Geometry check sheet. Reference: the model listing, model coordinates, mm. Face numbers are marked on the shaded views. A direction names the side the tool comes from. Give positions to 0.01 mm unless a question says otherwise; leave off trailing zeros. Write each loop counter-clockwise with the first axis right and the second up, starting at its lowest first coordinate (ties: lowest second). Pieces come first, ordered by that corner, then holes. Notation, with made-up numbers: M 35,-22.75 L 45,-22.75 A23 ccw 45,13.25 Z; hole C 16,53 d11. An arc over 180 degrees is marked long. One line per item, written item: value. Start each with the question number.
1. Cross-section at A-A on x = 0. Record the cut outline in (y, z), then the cut area to 3 significant figures.
2. Release check for a two-part mould opening along X. For the marked faces 4, 5 and 6 record: pulls with the +X half, pulls with the -X half, needs draft (parallel to the pull), parting line crosses it, or undercut.
3. Cross-section at B-B on z = 16. Record the cut outline in (x, y).
4. Tool access check on the marked faces 1, 2 and 3. Record the directions out of +Z, -Z, +X, -X, +Y, -Y that give a thin tool (end or side, any length) a straight path to the whole face; none if there is none.
5. Cross-section at D-D on z = 5.25. Record the cut outline in (x, y).
6. Gauge pin test, flat ends, axial feed: pin 1 (1.5 mm diameter, centred on y = -31.5, z = 5.5, fed in from -X); pin 2 (7.5 mm diameter, centred on x = -57, z = 7.5, fed in from +Y); pin 3 (1.5 mm diameter, centred on y = -32.5, z = 10.5, fed in from +X). Record the tip position at first contact, or that the pin passes through.
7. Cross-section at C-C on y = 0. Record the cut outline in (x, z).
8. Scan lines: line 1 (Z direction, x = 4, y = 7.5); line 2 (X direction, y = -45.5, z = 12.5); line 3 (X direction, y = -40, z = 1.25). Record each from-to range of solid material in increasing order.
from build123d import *

# Parameters (mm, degrees)
F0_R      = 11.6
F1_DEPTH  = 25.4
F2_R      = 11.6
F2_R_2    = 5.75
F3_DEPTH  = 16
F4_R      = 2.6054950693
F5_DEPTH  = 25
F6_DEPTH  = 13
F7_DEPTH  = 13
F8_DEPTH  = 25
F10_START = -13.2
F9_W      = 101.4740765095
F9_H      = 163.1420962512
F10_DEPTH = 15.6
F11_DEPTH = 19.8


with BuildPart() as f1:
    # F0 (on Top) → F1 (new body)
    with BuildSketch(Plane.XY):
        with BuildLine():
            Line((36.4474654198, -36.875538528), (21.8328172584, 7.2338157676))
            ThreePointArc((21.8328172584, 7.2338157676), (0, 23), (-21.8328172584, 7.2338157676))
            Line((-21.8328172584, 7.2338157676), (-36.4474654198, -36.875538528))
            ThreePointArc((-36.4474654198, -36.875538528), (-40.0855678291, -41.8375392315), (-45.9399946626, -43.7304012377))
            Line((-45.9399946626, -43.7304012377), (-60.6462528196, -43.7304012377))
            Line((-60.6462528196, -43.7304012377), (-60.6462528196, -50.8411786739))
            Line((-60.6462528196, -50.8411786739), (-25.3686927199, -50.8411786739))
            ThreePointArc((-25.3686927199, -50.8411786739), (0, -30.5358630094), (25.3686927199, -50.8411786739))
            Line((25.3686927199, -50.8411786739), (60.6462528196, -50.8411786739))
            Line((60.6462528196, -50.8411786739), (60.6462528196, -43.7304012377))
            Line((60.6462528196, -43.7304012377), (45.9399946626, -43.7304012377))
            ThreePointArc((45.9399946626, -43.7304012377), (40.0855678291, -41.8375392315), (36.4474654198, -36.875538528))
        make_face()
        Circle(F0_R, mode=Mode.SUBTRACT)
    extrude(amount=F1_DEPTH)

    # F2 (on face) → F3 (join)
    with BuildSketch(Plane.XY.offset(25.4)):
        Circle(F2_R)
        Circle(F2_R_2, mode=Mode.SUBTRACT)
    extrude(amount=-F3_DEPTH)

    # F4 (on face) → F5 (cut)
    with BuildSketch(Plane(origin=(0, -43.7304012377, 0), x_dir=(-1, 0, 0), z_dir=(0, 1, 0))):
        with Locations((-53.2931237411, 12.7)):
            Circle(F4_R)
        with Locations((53.2931237411, 12.7)):
            Circle(F4_R)
    extrude(amount=-F5_DEPTH, mode=Mode.SUBTRACT)

    # F2 (on face) → F6 (join)
    with BuildSketch(Plane.XY.offset(25.4)):
        with BuildLine():
            Line((-60.6462528196, -50.8411786739), (-25.3686927199, -50.8411786739))
            ThreePointArc((-25.3686927199, -50.8411786739), (0, -30.5358630094), (25.3686927199, -50.8411786739))
            Line((25.3686927199, -50.8411786739), (60.6462528196, -50.8411786739))
            Line((60.6462528196, -50.8411786739), (60.6462528196, -43.7304012377))
            Line((60.6462528196, -43.7304012377), (45.9399946626, -43.7304012377))
            ThreePointArc((45.9399946626, -43.7304012377), (40.0855678291, -41.8375392315), (36.4474654198, -36.875538528))
            Line((36.4474654198, -36.875538528), (21.8328172584, 7.2338157676))
            ThreePointArc((21.8328172584, 7.2338157676), (0, 23), (-21.8328172584, 7.2338157676))
            Line((-21.8328172584, 7.2338157676), (-36.4474654198, -36.875538528))
            ThreePointArc((-36.4474654198, -36.875538528), (-40.0855678291, -41.8375392315), (-45.9399946626, -43.7304012377))
            Line((-45.9399946626, -43.7304012377), (-60.6462528196, -43.7304012377))
            Line((-60.6462528196, -43.7304012377), (-60.6462528196, -50.8411786739))
        make_face()
        Circle(F2_R, mode=Mode.SUBTRACT)
    extrude(amount=F6_DEPTH)

    # F2 (on face) → F7 (join, through all)
    with BuildSketch(Plane.XY.offset(25.4)):
        Circle(F2_R)
        Circle(F2_R_2, mode=Mode.SUBTRACT)
    extrude(amount=F7_DEPTH)

    # F0 (on Top) → F8 (join)
    with BuildSketch(Plane.XY):
        with BuildLine():
            Line((36.4474654198, -36.875538528), (21.8328172584, 7.2338157676))
            ThreePointArc((21.8328172584, 7.2338157676), (0, 23), (-21.8328172584, 7.2338157676))
            Line((-21.8328172584, 7.2338157676), (-36.4474654198, -36.875538528))
            ThreePointArc((-36.4474654198, -36.875538528), (-40.0855678291, -41.8375392315), (-45.9399946626, -43.7304012377))
            Line((-45.9399946626, -43.7304012377), (-60.6462528196, -43.7304012377))
            Line((-60.6462528196, -43.7304012377), (-60.6462528196, -50.8411786739))
            Line((-60.6462528196, -50.8411786739), (-25.3686927199, -50.8411786739))
            ThreePointArc((-25.3686927199, -50.8411786739), (0, -30.5358630094), (25.3686927199, -50.8411786739))
            Line((25.3686927199, -50.8411786739), (60.6462528196, -50.8411786739))
            Line((60.6462528196, -50.8411786739), (60.6462528196, -43.7304012377))
            Line((60.6462528196, -43.7304012377), (45.9399946626, -43.7304012377))
            ThreePointArc((45.9399946626, -43.7304012377), (40.0855678291, -41.8375392315), (36.4474654198, -36.875538528))
        make_face()
        Circle(F0_R, mode=Mode.SUBTRACT)
    extrude(amount=F8_DEPTH)

    # F9 (on Front) → F10 (cut)
    with BuildSketch(Plane.XZ.offset(F10_START)):
        with Locations((-7.8580155969, 21.2894622236)):
            Rectangle(F9_W, F9_H)
    extrude(amount=-F10_DEPTH, mode=Mode.SUBTRACT)

    # F11 (cut): a face of the model
    f11_faces = [f1.faces().sort_by_distance(p)[0] for p in [
        (0, -21.0137412442, 38.4),
    ]]
    extrude(f11_faces, amount=-F11_DEPTH, mode=Mode.SUBTRACT)


solid = f1.part
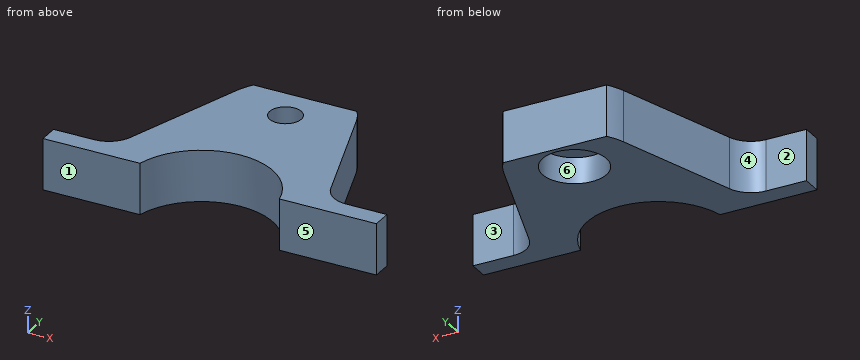
Report:
1. outline: M -30.54,0 L -11.6,0 L -11.6,9.4 L -5.75,9.4 L -5.75,18.6 L -30.54,18.6 Z; M 5.75,9.4 L 11.6,9.4 L 11.6,0 L 13.2,0 L 13.2,18.6 L 5.75,18.6 Z
1. area: 490 mm^2
2. face 4: pulls with the -X half
2. face 5: needs draft
2. face 6: undercut
3. outline: M -60.65,-50.84 L -25.37,-50.84 A26 cw 25.37,-50.84 L 60.65,-50.84 L 60.65,-43.73 L 45.94,-43.73 A10 cw 36.45,-36.88 L 21.83,7.23 A23 ccw 18.84,13.2 L -18.84,13.2 A23 ccw -21.83,7.23 L -36.45,-36.88 A10 cw -45.94,-43.73 L -60.65,-43.73 Z; hole C 0,0 d11.5
4. face 1: +Z, -Z, +X, -X, -Y
4. face 2: +Z, -Z, -X, +Y
4. face 3: +Z, -Z, +X, +Y
5. outline: M -60.65,-50.84 L -25.37,-50.84 A26 cw 25.37,-50.84 L 60.65,-50.84 L 60.65,-43.73 L 45.94,-43.73 A10 cw 36.45,-36.88 L 21.83,7.23 A23 ccw 18.84,13.2 L -18.84,13.2 A23 ccw -21.83,7.23 L -36.45,-36.88 A10 cw -45.94,-43.73 L -60.65,-43.73 Z; hole C 0,0 d23.2
6. pin 1: stops at x = -34.91
6. pin 2: stops at y = -43.73
6. pin 3: stops at x = 35.25
7. outline: M -24.23,0 L -11.6,0 L -11.6,9.4 L -5.75,9.4 L -5.75,18.6 L -24.23,18.6 Z; M 5.75,9.4 L 11.6,9.4 L 11.6,0 L 24.23,0 L 24.23,18.6 L 5.75,18.6 Z
8. line 1: z = 9.4 to 18.6
8. line 2: x = -60.65 to -23.54, 23.54 to 60.65
8. line 3: x = -38.15 to -20.06, 20.06 to 38.15
